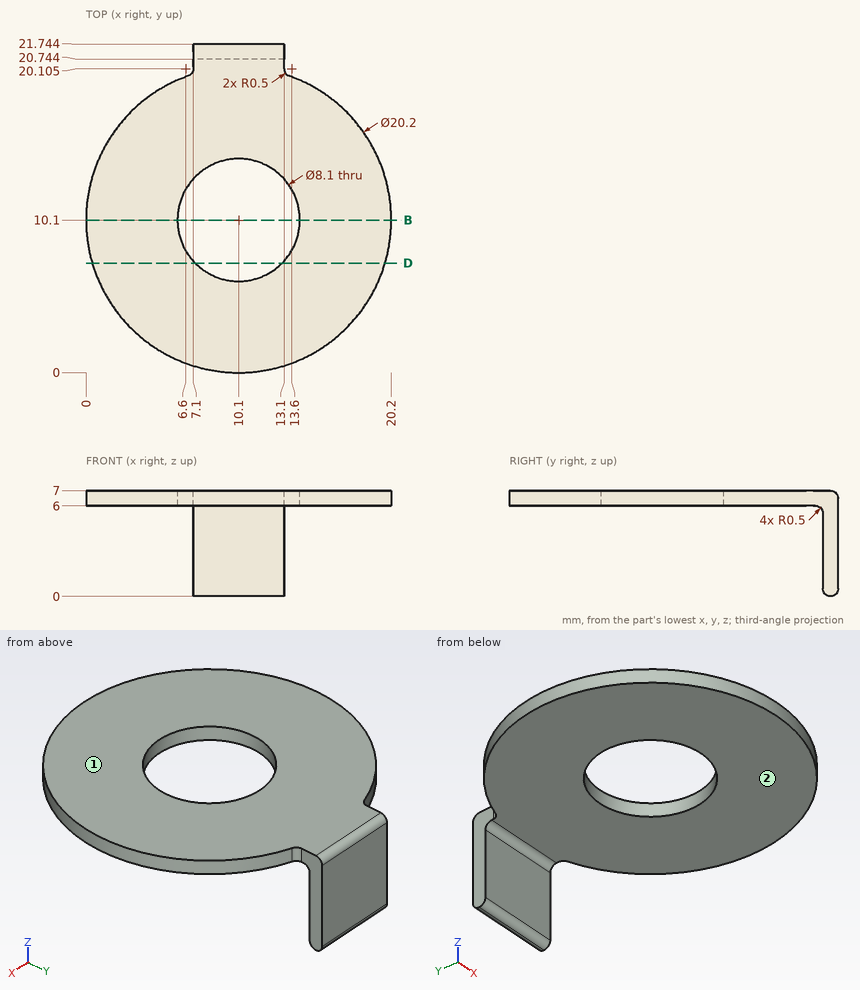
Here's the drawing with two shaded views (mm, measured from the low corner). I have some questions. A direction names the side the tool comes from. Give positions to 0.01 mm unless a question says otherwise; leave off trailing zeros. Order: outer loops, then holes, each group sorted by start corner. A loop starts at its lowest first (then second) coordinate and runs counter-clockwise, first axis right, second up. Notation, with made-up numbers: (9.25, 67) - (49.25, 67) arc R22 cw to (49.25, 79) - close; hole circle Ø9 at (-5.5, -9.75). An arc over 180 degrees is marked (long way). Use a Markdown table: item, result. Add a question column.
Q1. If we section it at D-D on y = 7.25: Write out the boundary of the cut face in (x, z).
Q2. Please list where these lines run through material, in increasing order: line 1 along Z through (x, y) = (2.5, 7.25); line 2 along Y through (x, z) = (11.5, 1.5) (1 decimal); line 3 along Y through (x, z) = (15.25, 6.25).
Q3. On a 3-axis mill with a long thin cutter (end or side, diameter ignored), from which of +Z, -Z, +X, -X, +Y, -Y can I reach the whole of each face in a straight line? I mean the marked faces 1 and 2. Say none if no direction works.
Q4. If we section it at B-B on y = 10.1: Write out the boundary of the cut face in (x, z), plus the area to 3 significant figures.
Q5. I'm going to push flat-ended pins straight in: pin 1 (2 mm diameter, centred on x = 13, z = 1.5, fed in from -Y); pin 2 (2 mm diameter, centred on x = 5.5, y = 8, fed in from -Z); pin 3 (1.3 mm diameter, centred on y = 21, z = 4, fed in from -X); pin 4 (4 mm diameter, centred on x = 4.5, z = 2, fed in from +Y). Where does each tip first touch, or does it pass through?
Answers follow:
| question | item | result |
|---|---|---|
| 1 | outline | (0.41, 6) - (7.22, 6) - (7.22, 7) - (0.41, 7) - close; (12.98, 6) - (19.79, 6) - (19.79, 7) - (12.98, 7) - close |
| 2 | line 1 | z = 6 to 7 |
| 2 | line 2 | y = 20.7 to 21.7 |
| 2 | line 3 | y = 1.41 to 18.79 |
| 3 | face 1 | +Z, +X, -X, +Y, -Y |
| 3 | face 2 | -Z, +X, -X, -Y |
| 4 | outline | (0, 6) - (6.05, 6) - (6.05, 7) - (0, 7) - close; (14.15, 6) - (20.2, 6) - (20.2, 7) - (14.15, 7) - close |
| 4 | area | 12.1 mm^2 |
| 5 | pin 1 | stops at y = 20.74 |
| 5 | pin 2 | stops at z = 6 |
| 5 | pin 3 | stops at x = 7.1 |
| 5 | pin 4 | passes through |
